Source: CAD feature listing. Evaluate the final solid. Frame: model axes, mm. A direction names the side the tool comes from. Coordinates: 2 decimals unless noted, no trailing zeros. Order: outer loops, then holes, each group sorted by start corner. A loop starts at its lowest first (then second) coordinate and runs counter-clockwise, first axis right, second up. Notation, with made-up numbers: (-32.75, 47) - (10.25, 47) arc R15 ccw to (10.25, 54) - close; hole circle Ø9 at (14, 86.5). An arc over 180 degrees is marked (long way). One line per question, with ' | ' between items. Start each with the question number.
(1) Draft query along X for faces 1 (the flat face through (-1, 12.7, 3)), 2 (the cylindrical face through (-2.404, 1.282, 3.135)), 3 (the cylindrical face through (0.1, 6.3, -2.9)). Return one class per face: +X half, -X half, draft (parallel to the pull), parting line (faces both ways), or undercut.
(2) Line query: line 1 along X through (y, z) = (12.25, 1.75); line 2 along Z through (x, y) = (-0.75, 4.75); line 3 along X through (y, z) = (8, 0). Output: solid intervals per line, ascending.
(3) Section A-A (x = 0). Return the cut outline in (y, z), then the cut area to 3 significant figures.
(4) Contact query for flat-ended pins moving along their axis: P1, Ø3, axis at x = 0.5, y = 7.5, coming from the -Z side; P2, Ø1.5, axis at x = -0.5, z = -0.5, coming from the -Y side; P3, Ø2, axis at x = 2, y = 1.5, coming from the -Z side. Output: stop coordinate, or through.
(5) Access query for faces 4 (the flat face through (3, 0, -1)), 5 (the flat face through (0, 8, -4)). Directions: +Z, -Z, +X, -X, +Y, -Y. A direction counts if a zero-diameter tool reaches every point of the face in a straight line with its end or side. Return the directions, or none.
from build123d import *

# Parameters (mm, degrees)
ESQUISSE1_R             = 4.35
ESQUISSE1_R_2           = 2.9
BOSS_EXTRU_1_DEPTH      = 12.7
ESQUISSE2_OUTSIDE_W     = 14.236
ESQUISSE2_OUTSIDE_H     = 14.236
ESQUISSE2_OUTSIDE_R     = 3.95
ENL_V_MAT_EXTRU_1_DEPTH = 2
CHANFREIN1_SIZE         = 1
ENL_V_MAT_EXTRU_2_DEPTH = 15.111520117


with BuildPart() as part:
    # Esquisse1 → Boss.-Extru.1 (new body)
    with BuildSketch(Plane(origin=(0, 0, 0), x_dir=(1, 0, 0), z_dir=(0, 1, 0))):
        with Locations(Location((0, 0, 0), (0, 0, 270))):
            Circle(ESQUISSE1_R)
        with Locations(Location((0, 0, 0), (0, 0, 270))):
            Circle(ESQUISSE1_R_2, mode=Mode.SUBTRACT)
    extrude(amount=BOSS_EXTRU_1_DEPTH)

    # Esquisse2 outside → Enlèv. mat.-Extru.1 (cut)
    with BuildSketch(Plane.XZ):
        Rectangle(ESQUISSE2_OUTSIDE_W, ESQUISSE2_OUTSIDE_H)
        with Locations(Location((0, 0, 0), (0, 0, 270))):
            Circle(ESQUISSE2_OUTSIDE_R, mode=Mode.SUBTRACT)
    extrude(amount=-ENL_V_MAT_EXTRU_1_DEPTH, mode=Mode.SUBTRACT)

    # Chanfrein1
    # the kernel refuses this chamfer: 1 mm, written as the material it takes off along each edge
    with BuildSketch(Plane(origin=(0, 2, 0), x_dir=(0, 0, 1), z_dir=(1, 0, 0))) as chanfrein1_piece_1_section:
        Polygon((4.35, -CHANFREIN1_SIZE), (4.35 - CHANFREIN1_SIZE, 0), (4.35, 0), align=None)
    chanfrein1_piece_1 = revolve(axis=Axis((0, 2, 0), (0, -1, 0)), mode=Mode.PRIVATE)
    chanfrein1_piece_1 = chanfrein1_piece_1 - Plane(origin=(0, 2.799298708, 0), x_dir=(0, 0, -1), z_dir=(0, -1, 0)) * Cylinder(3.95, 18, mode=Mode.PRIVATE)
    add(chanfrein1_piece_1, mode=Mode.SUBTRACT)

    # Esquisse3 → Enlèv. mat.-Extru.2 (cut, through all)
    with BuildSketch(Plane(origin=(0, 12.7, 0), x_dir=(1, 0, 0), z_dir=(0, 1, 0))):
        Polygon((1, 4.856888804), (-1, 4.856888804), (-0.4, 4), (0.4, 4), align=None)
        Polygon((2.889020106, 4.030252062), (1.06192919, 4.843725348), (1.261528389, 3.816876488), (1.992364755, 3.491487173), align=None)
        Polygon((4.278502389, 2.506748125), (2.940241176, 3.993037776), (2.704927059, 2.973780356), (3.240231544, 2.379264495), align=None)
        Polygon((4.92819274, 0.549804664), (4.310158752, 2.451917697), (3.680619267, 1.616490584), (3.927832863, 0.855645371), align=None)
        Polygon((4.725753796, -1.502205018), (4.934810722, 0.486838772), (4.019898967, -0.020305095), (3.936276196, -0.815922611), align=None)
        Polygon((3.706189088, -3.294469806), (4.706189088, -1.562418998), (3.664101615, -1.653589838), (3.264101615, -2.346410162), align=None)
        Polygon((2.045790617, -4.517090835), (3.663824605, -3.34152033), (2.674747807, -3.000953877), (2.027534211, -3.471182078), align=None)
        Polygon((0.031656363, -4.958665822), (1.987951564, -4.54284244), (1.222905804, -3.829425727), (0.440387723, -3.995755079), align=None)
        Polygon((-1.987951564, -4.54284244), (-0.031656363, -4.958665822), (-0.440387723, -3.995755079), (-1.222905804, -3.829425727), align=None)
        Polygon((-3.663824605, -3.34152033), (-2.045790617, -4.517090835), (-2.027534211, -3.471182078), (-2.674747807, -3.000953877), align=None)
        Polygon((-4.706189088, -1.562418998), (-3.706189088, -3.294469806), (-3.264101615, -2.346410162), (-3.664101615, -1.653589838), align=None)
        Polygon((-4.934810722, 0.486838772), (-4.725753796, -1.502205018), (-3.936276196, -0.815922611), (-4.019898967, -0.020305095), align=None)
        Polygon((-4.310158752, 2.451917697), (-4.92819274, 0.549804664), (-3.927832863, 0.855645371), (-3.680619267, 1.616490584), align=None)
        Polygon((-2.940241176, 3.993037776), (-4.278502389, 2.506748125), (-3.240231544, 2.379264495), (-2.704927059, 2.973780356), align=None)
        Polygon((-1.06192919, 4.843725348), (-2.889020106, 4.030252062), (-1.992364755, 3.491487173), (-1.261528389, 3.816876488), align=None)
    extrude(amount=-ENL_V_MAT_EXTRU_2_DEPTH, mode=Mode.SUBTRACT)


solid = part.part
Response values:
1) face 1: draft | face 2: parting line | face 3: undercut
2) line 1: x = -3.61 to -2.31, 2.31 to 3.61 | line 2: z = -4.28 to -2.8, 2.8 to 3.93 | line 3: x = -4.06 to -2.9, 2.9 to 4.06
3) outline: (0, -3.95) - (2.6, -3.95) - (2.65, -4) - (12.7, -4) - (12.7, -2.9) - (0, -2.9) - close; (0, 2.9) - (12.7, 2.9) - (12.7, 4.35) - (3, 4.35) - (2.6, 3.95) - (0, 3.95) - close | area: 31.1 mm²
4) P1: stops at z = -4.31 | P2: passes through | P3: stops at z = -3.82
5) face 4: +Z, -Z, +X, -X, -Y | face 5: -Z, +Y, -Y
